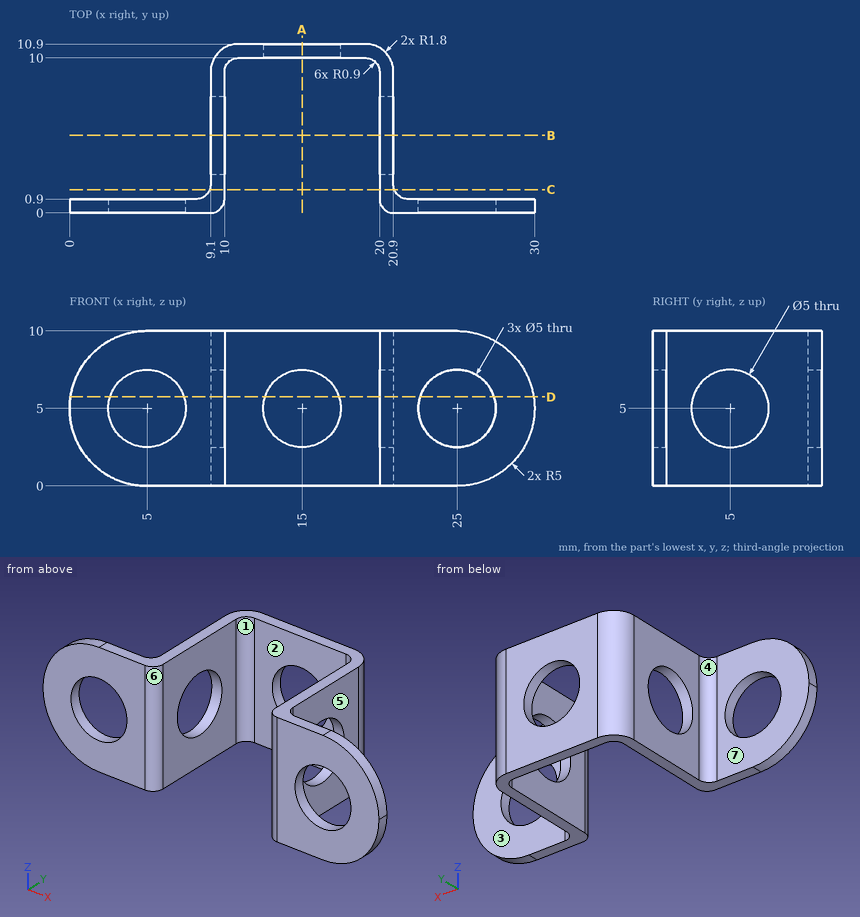
Could you check a few things on this drawing? It's one solid part, dimensions in mm from its lowest x, y, z. A direction names the side the tool comes from. Round coordinates to 2 decimals unless told otherwise and drop trailing zeros. Order: outer loops, then holes, each group sorted by start corner. A loop starts at its lowest first (then second) coordinate and runs counter-clockwise, first axis right, second up. Notation, with made-up numbers: (49.25, 2) -> (61.25, 2) arc R19 ccw to (61.25, 17) -> close; hole circle Ø7 at (-34.5, -32). An arc over 180 degrees is marked (long way). One line per question, with ' | ' between items.
Q1. If we section it at D-D on z = 5.75: Give the number of separate pieces and of enclosed holes in the cut face, plus the area to 3 significant figures.
Computed values:
separate pieces: 6 | enclosed holes: 0 | area: 22.4 mm²
Q2. We'd pull the mould along X, two halves only. Please class the marked faces 1, 2, 3 and 4: released by +X, released by -X, zero draft, split by the parting line, or undercut.
Computed values:
face 1: undercut | face 2: undercut | face 3: zero draft | face 4: released by -X
Q3. If I drill on line 1 (X direction, y = 3.25, z = 2.25); line 2 (Z direction, x = 9.6, y = 5); line 3 (Y direction, x = 28, z = 6.5), over which ranges is the centre line in solid material (lowest first)? Write a range as from..to.
Computed values:
line 1: 9.1..10, 20..20.9 | line 2: 0..2.5, 7.5..10 | line 3: 0..0.9
Q4. Which directions (+Z, -Z, +X, -X, +Y, -Y) give clear straight access to the entire face, cutting with the end or side of a thin tool? Please do the marked faces 5, 6 and 7.
Computed values:
face 5: +Z, -Z, +X, +Y | face 6: +Z, -Z, -Y | face 7: +Z, -Z, -X, +Y
Q5. I'm going to push flat-ended pins straight in: pin 1 (1 mm diameter, centred on x = 14.5, z = 4, fed in from +Y); pin 2 (2.5 mm diameter, centred on y = 7, z = 3.5, fed in from +X); pin 3 (4 mm diameter, centred on y = 4, z = 6.5, fed in from -X); pin 4 (6 mm diameter, centred on y = 4.5, z = 6, fed in from -X). Where does each tip first touch, or does it pass through?
Computed values:
pin 1: through | pin 2: x = 20.9 | pin 3: x = 9.1 | pin 4: x = 9.05
Q6. If we section it at A-A on x = 15: Write out the boundary of the cut face in (y, z), plus the area to 3 significant figures.
Computed values:
outline: (10, 0) -> (10.9, 0) -> (10.9, 2.5) -> (10, 2.5) -> close; (10, 7.5) -> (10.9, 7.5) -> (10.9, 10) -> (10, 10) -> close | area: 4.50 mm²
Q7. If we section it at B-B on y = 5: Write out the boundary of the cut face in (x, z).
Computed values:
outline: (9.1, 0) -> (10, 0) -> (10, 2.5) -> (9.1, 2.5) -> close; (9.1, 7.5) -> (10, 7.5) -> (10, 10) -> (9.1, 10) -> close; (20, 0) -> (20.9, 0) -> (20.9, 2.5) -> (20, 2.5) -> close; (20, 7.5) -> (20.9, 7.5) -> (20.9, 10) -> (20, 10) -> close
Q8. If we section it at C-C on y = 1.5: Write out the boundary of the cut face in (x, z), plus the area to 3 significant figures.
Computed values:
outline: (9.05, 0) -> (10, 0) -> (10, 10) -> (9.05, 10) -> close; (20, 0) -> (20.95, 0) -> (20.95, 10) -> (20, 10) -> close | area: 19.0 mm²
